```python
from build123d import *

# Parameters (mm, degrees)
SKETCH_1_W          = 62
SKETCH_1_H          = 8
EXTRUDE_1_DEPTH     = 2
SKETCH_2_R          = 12
SKETCH_2_R_2        = 1.7
EXTRUDE_2_DEPTH     = 2
EXTRUDE_START       = 2
SKETCH_3_R          = 10
SKETCH_3_R_2        = 1.7
EXTRUDE_3_DEPTH     = 2.2
EXTRUDE_START_2     = 13
SKETCH_4_W          = 20
SKETCH_4_H          = 7
EXTRUDE_4_DEPTH     = 2
SKETCH_5_R          = 15
SKETCH_5_R_2        = 1.6
EXTRUDE_5_DEPTH     = 2
EXTRUDE_START_3     = -3.5
SKETCH_6_W          = 74
SKETCH_6_H          = 15
EXTRUDE_6_DEPTH     = 7
SKETCH_7_W          = 13.866896788
SKETCH_7_H          = 9.192033752
CUT_EXTRUDE_1_DEPTH = 10
SKETCH_8_W          = 10
SKETCH_8_H          = 24
CUT_EXTRUDE_2_DEPTH = 10


with BuildPart() as part:
    # Sketch 1 → Extrude 1 (new body)
    with BuildSketch(Plane(origin=(0, 0, 0), x_dir=(1, 0, 0), z_dir=(0, 1, 0))):
        with Locations((31, 0)):
            Rectangle(SKETCH_1_W, SKETCH_1_H)
    extrude(amount=EXTRUDE_1_DEPTH)

    # Sketch 2 → Extrude 2 (add)
    with BuildSketch(Plane(origin=(0, 0, 0), x_dir=(1, 0, 0), z_dir=(0, 1, 0))):
        Circle(SKETCH_2_R)
        with Locations(Location((0, -7, 0), (0, 0, 270))):
            Circle(SKETCH_2_R_2, mode=Mode.SUBTRACT)
        with Locations(Location((0, 7, 0), (0, 0, 270))):
            Circle(SKETCH_2_R_2, mode=Mode.SUBTRACT)
    extrude(amount=EXTRUDE_2_DEPTH)

    # Sketch 3 → Extrude 3 (add)
    with BuildSketch(Plane(origin=(0, 0, 0), x_dir=(1, 0, 0), z_dir=(0, 1, 0)).offset(EXTRUDE_START)):
        with Locations(Location((0, 0, 0), (0, 0, 270))):
            Circle(SKETCH_3_R)
        with Locations(Location((0, -7, 0), (0, 0, 270))):
            Circle(SKETCH_3_R_2, mode=Mode.SUBTRACT)
        with Locations(Location((0, 7, 0), (0, 0, 270))):
            Circle(SKETCH_3_R_2, mode=Mode.SUBTRACT)
    extrude(amount=EXTRUDE_3_DEPTH)



with BuildPart() as body_2:
    # Sketch 4 → Extrude 4 (new body)
    with BuildSketch(Plane(origin=(0, 0, 0), x_dir=(1, 0, 0), z_dir=(0, 1, 0)).offset(EXTRUDE_START_2)):
        Rectangle(SKETCH_4_W, SKETCH_4_H)
    extrude(amount=EXTRUDE_4_DEPTH)


with BuildPart() as body_3:
    # Sketch 5 → Extrude 5 (new body)
    with BuildSketch(Plane(origin=(0, 0, 0), x_dir=(1, 0, 0), z_dir=(0, 1, 0))):
        with Locations(Location((78, 0, 0), (0, 0, 270))):
            Circle(SKETCH_5_R)
        with Locations(Location((70, -9.5, 0), (0, 0, 270))):
            Circle(SKETCH_5_R_2, mode=Mode.SUBTRACT)
        with Locations(Location((70, 9.5, 0), (0, 0, 270))):
            Circle(SKETCH_5_R_2, mode=Mode.SUBTRACT)
        with Locations(Location((86, -9.5, 0), (0, 0, 270))):
            Circle(SKETCH_5_R_2, mode=Mode.SUBTRACT)
        with Locations(Location((86, 9.5, 0), (0, 0, 270))):
            Circle(SKETCH_5_R_2, mode=Mode.SUBTRACT)
    extrude(amount=EXTRUDE_5_DEPTH)


with BuildPart() as part_1:
    add(part.part)

    add(body_2.part)  # Extrude 6 merges body 2

    add(body_3.part)  # Extrude 6 merges body 3
    # Sketch 6 → Extrude 6 (add)
    with BuildSketch(Plane.XY.offset(EXTRUDE_START_3)):
        with Locations((37, 7.5)):
            Rectangle(SKETCH_6_W, SKETCH_6_H)
        Polygon((5, 2), (18, 2), (15, 13), (8, 13), align=None, mode=Mode.SUBTRACT)
        Polygon((18, 13), (31, 13), (28, 2), (21, 2), align=None, mode=Mode.SUBTRACT)
        Polygon((31, 2), (44, 2), (41, 13), (34, 13), align=None, mode=Mode.SUBTRACT)
        Polygon((44, 13), (57, 13), (54, 2), (47, 2), align=None, mode=Mode.SUBTRACT)
        Polygon((57, 2), (71, 2), (68, 13), (60, 13), align=None, mode=Mode.SUBTRACT)
    extrude(amount=EXTRUDE_6_DEPTH)

    # Sketch 7 → Cut-Extrude 1 (cut)
    with BuildSketch(Plane.XZ.offset(-13)):
        with Locations((-6.933448394, 0.107084937)):
            Rectangle(SKETCH_7_W, SKETCH_7_H)
    extrude(amount=-CUT_EXTRUDE_1_DEPTH, mode=Mode.SUBTRACT)

    # Sketch 8 → Cut-Extrude 2 (cut)
    with BuildSketch(Plane(origin=(0, 4.2, 0), x_dir=(1, 0, 0), z_dir=(0, 1, 0))):
        with Locations((-10, 0)):
            Rectangle(SKETCH_8_W, SKETCH_8_H)
    extrude(amount=-CUT_EXTRUDE_2_DEPTH, mode=Mode.SUBTRACT)


solid = part_1.part
```
Design review of the part built by this model. Coordinates are the model's own, in mm. A direction names the side the tool comes from. Round coordinates to 2 decimals unless told otherwise and drop trailing zeros. Order: outer loops, then holes, each group sorted by start corner. A loop starts at its lowest first (then second) coordinate and runs counter-clockwise, first axis right, second up. Notation, with made-up numbers: (-8.5, -6) - (0.5, -6) arc R23 ccw to (0.5, 30) - close; hole circle Ø4 at (-17, 4.5). An arc over 180 degrees is marked (long way). One line per question, with ' | ' between items.
Item 1: For P1, Ø1, axis at x = 49, y = 1.5, coming from the +Z side; P2, Ø5, axis at x = 70, z = 9.5, coming from the +Y side; P3, Ø2, axis at x = 24, y = 1, coming from the -Z side, all flat-tipped, find the tip position at first contact; note any pin that passes through.
Checks:
P1: z = 4 | P2: y = 2 | P3: z = -4
Item 2: Take a section at B-B, the plane z = -6.75. Write out the cut boundary in (x, y).
Checks:
outline: (-5, 0) - (-1.68, 0) - (-1.68, 4.2) - (-5, 4.2) - close; (1.68, 0) - (9.92, 0) - (9.92, 2) - (7.38, 2) - (7.38, 4.2) - (1.68, 4.2) - close; (64.6, 0) - (91.4, 0) - (91.4, 2) - (64.6, 2) - close
Item 3: Take a section at D-D, the plane x = 70. Write out the cut boundary in (y, z), then the cut area to 3 significant figures.
Checks:
outline: (0, -12.69) - (2, -12.69) - (2, -11.1) - (0, -11.1) - close; (0, -7.9) - (2, -7.9) - (2, 7.9) - (0, 7.9) - close; (0, 11.1) - (2, 11.1) - (2, 12.69) - (0, 12.69) - close; (5.67, -3.5) - (15, -3.5) - (15, 3.5) - (5.67, 3.5) - close | area: 103 mm²
Item 4: Wall thickness on line 1 (Y direction, x = 52.5, z = 1.25); line 2 (Z direction, x = 1.5, y = 3.5); line 3 (X direction, y = 1.95, z = 7): over which ranges is each line inside the solid? List them lowest first. Write a range as [from, to].
Checks:
line 1: [0, 2], [13, 15] | line 2: [-9.89, -7.8], [-6.2, 6.2], [7.8, 9.89] | line 3: [-5, -1.7], [1.7, 9.75], [64.73, 91.27]
Item 5: Take a section at A-A, the plane x = 19.5. Write out the cut boundary in (y, z), then the cut area to 3 significant figures.
Checks:
outline: (0, -4) - (2, -4) - (2, -3.5) - (7.5, -3.5) - (7.5, 3.5) - (2, 3.5) - (2, 4) - (0, 4) - close; (13, -3.5) - (15, -3.5) - (15, 3.5) - (13, 3.5) - close | area: 68.5 mm²
Item 6: Draft analysis for pull direction Z (two halves, no side actions). For faces 1 (the face through (4.8, 1, -11)), 2 (the face through (50, 13, 0)), 3 (the face through (87.586, 0.986, 9.292)), state which applies: +Z half, -Z half, draft (parallel to the pull), parting line (faces both ways), or undercut.
Checks:
face 1: -Z half | face 2: draft | face 3: undercut
Item 7: Machinability: for faces 4 (the face through (74, 8, 0)), 5 (the face through (36, 1, 4)), 6 (the face through (32.52, 7.58, -0.05)), which of the approach directions +Z, -Z, +X, -X, +Y, -Y give a long, thin tool a straight path to every point of the face, cutting with its end or side? Answer none if there is none.
Checks:
face 4: +Z, -Z, +X, +Y | face 5: +Z, +Y, -Y | face 6: +Z, -Z
Item 8: Take a section at C-C, the plane y = 10. Write out the cut boundary in (x, z).
Checks:
outline: (0, -3.5) - (7.18, -3.5) - (7.18, 3.5) - (0, 3.5) - close; (15.82, -3.5) - (18.82, -3.5) - (18.82, 3.5) - (15.82, 3.5) - close; (30.18, -3.5) - (33.18, -3.5) - (33.18, 3.5) - (30.18, 3.5) - close; (41.82, -3.5) - (44.82, -3.5) - (44.82, 3.5) - (41.82, 3.5) - close; (56.18, -3.5) - (59.18, -3.5) - (59.18, 3.5) - (56.18, 3.5) - close; (68.82, -3.5) - (74, -3.5) - (74, 3.5) - (68.82, 3.5) - close
